Read the model definition and answer for the solid it produces. Units are mm, in the model's axes. Coordinates: 2 decimals unless noted, no trailing zeros. Write each loop counter-clockwise with the first axis right and the second up, starting at its lowest first coordinate (ties: lowest second). Pieces come first, ordered by that corner, then holes. Notation, with made-up numbers: (16.5, 72.5) -> (66.5, 72.5) arc R25 cw to (66.5, 106.5) -> close; hole circle Ø5 at (-1, 65.5). An arc over 180 degrees is marked (long way). Write item = value, one per line. Start each with the question number.
1) Section D-D (z = -105) is taken. Determine the outline of the cut face in (x, y), plus the area to 3 significant figures.
2) Find the intervals of material crossed by line 1 along Z through (x, y) = (-8, -2.05); line 2 along X through (y, z) = (-4.5, -12); line 3 along Z through (x, y) = (-124, -2.65), in increasing order. Write a range as from..to.
3) Section C-C (z = 33.5) is taken. Determine the outline of the cut face in (x, y).
4) Section B-B (z = -54.5) is taken. Determine the outline of the cut face in (x, y), plus the area to 3 significant figures.
5) Flat-ended cylindrical pins translate along their axes: pin 1 Ø1 at (x, y) = (-46, -2.5) entering from +Z; pin 2 Ø1 at (y, z) = (-3, -18) entering from -X. Find the tip coordinate at first contact, or state that the pin passes through.
6) Section A-A (y = -2.7) is taken. Count the separate pieces of the cut face and the enclosed holes in it, plus the area to 3 significant figures.
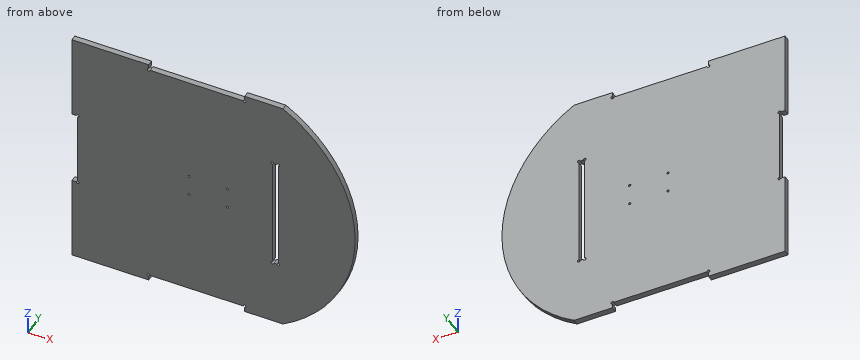
from build123d import *

# Parameters (mm, degrees)
BOSS_EXTRUDE1_DEPTH       = 6
M2_CLEARANCE_HOLE1_D      = 2.4
CUT_EXTRUDE1_REACH        = 212.276
SKETCH4_W                 = 6.1
SKETCH4_H                 = 120.1
SKETCH4_W_2               = 100.1
SKETCH4_H_2               = 6.1
SKETCH4_H_3               = 80.1
F_3_0MM_DOWEL_HOLE1_D     = 3
F_3_0MM_DOWEL_HOLE1_DEPTH = 6


with BuildPart() as part:
    # Sketch1 → Boss-Extrude1 (new body)
    with BuildSketch(Plane(origin=(0, 0, 0), x_dir=(1, 0, 0), z_dir=(0, 1, 0))):
        with BuildLine():
            Line((-130, 130), (90, 130))
            ThreePointArc((90, 130), (165.166852265, 0), (90, -130))
            Line((90, -130), (-130, -130))
            Line((-130, -130), (-130, 130))
        make_face()
    extrude(amount=-BOSS_EXTRUDE1_DEPTH)

    # M2 Clearance Hole1 (through all)
    with Locations(Plane(origin=(0, -6, 0), x_dir=(-1, 0, 0), z_dir=(0, -1, 0))):
        with Locations((-32, -11), (-32, 11), (8, -11), (8, 11)):
            Hole(M2_CLEARANCE_HOLE1_D / 2)

    # Sketch4 → Cut-Extrude1 (cut, up to next)
    with BuildSketch(Plane.XZ.offset(6), mode=Mode.PRIVATE) as cut_extrude1_sk1:
        with Locations((82, 0)):
            Rectangle(SKETCH4_W, SKETCH4_H)
    cut_extrude1_tool1 = extrude(cut_extrude1_sk1.sketch, amount=-CUT_EXTRUDE1_REACH, mode=Mode.PRIVATE) & part.part
    # Sketch4 → Cut-Extrude1 (cut, up to next)
    with BuildSketch(Plane.XZ.offset(6), mode=Mode.PRIVATE) as cut_extrude1_sk2:
        with Locations((0, -127)):
            Rectangle(SKETCH4_W_2, SKETCH4_H_2)
    cut_extrude1_tool2 = extrude(cut_extrude1_sk2.sketch, amount=-CUT_EXTRUDE1_REACH, mode=Mode.PRIVATE) & part.part
    # Sketch4 → Cut-Extrude1 (cut, up to next)
    with BuildSketch(Plane.XZ.offset(6), mode=Mode.PRIVATE) as cut_extrude1_sk3:
        with Locations((0, 127)):
            Rectangle(SKETCH4_W_2, SKETCH4_H_2)
    cut_extrude1_tool3 = extrude(cut_extrude1_sk3.sketch, amount=-CUT_EXTRUDE1_REACH, mode=Mode.PRIVATE) & part.part
    # Sketch4 → Cut-Extrude1 (cut, up to next)
    with BuildSketch(Plane.XZ.offset(6), mode=Mode.PRIVATE) as cut_extrude1_sk4:
        with Locations((-127, 0)):
            Rectangle(SKETCH4_W, SKETCH4_H_3)
    cut_extrude1_tool4 = extrude(cut_extrude1_sk4.sketch, amount=-CUT_EXTRUDE1_REACH, mode=Mode.PRIVATE) & part.part
    add(cut_extrude1_tool1.solids().sort_by_distance((82, -6, 0))[0], mode=Mode.SUBTRACT)
    add(cut_extrude1_tool2.solids().sort_by_distance((0, -6, -127))[0], mode=Mode.SUBTRACT)
    add(cut_extrude1_tool3.solids().sort_by_distance((0, -6, 127))[0], mode=Mode.SUBTRACT)
    add(cut_extrude1_tool4.solids().sort_by_distance((-127, -6, 0))[0], mode=Mode.SUBTRACT)

    # Ø3.0mm Dowel Hole1
    with Locations(Plane(origin=(0, -6, 0), x_dir=(-1, 0, 0), z_dir=(0, -1, 0))):
        with Locations((-85, 60), (-79, 60), (-78.95, -60.05), (-85, -60), (124, 40), (123.95, -40.05), (50.05, -123.95), (-50, -124), (-50.05, 123.95), (50.05, 123.95)):
            Hole(F_3_0MM_DOWEL_HOLE1_D / 2, depth=F_3_0MM_DOWEL_HOLE1_DEPTH)


solid = part.part
Answer key:
q1.outline = (-130, -6) -> (122.29, -6) -> (122.29, 0) -> (-130, 0) -> close
q1.area = 1,510 mm^2
q2.line_1 = -123.95..-12.2, -9.8..9.8, 12.2..123.95
q2.line_2 = -123.95..-8.66, -7.34..31.34, 32.66..78.95, 85.05..164.69
q2.line_3 = -130..-41.5, 41.55..130
q3.outline = (-123.95, -6) -> (78.95, -6) -> (78.95, 0) -> (-123.95, 0) -> close; (85.05, -6) -> (161.38, -6) -> (161.38, 0) -> (85.05, 0) -> close
q4.outline = (-130, -6) -> (78.95, -6) -> (78.95, 0) -> (-130, 0) -> close; (85.05, -6) -> (154.92, -6) -> (154.92, 0) -> (85.05, 0) -> close
q4.area = 1,670 mm^2
q5.pin_1 = 123.95
q5.pin_2 = -123.95
q6.separate_pieces = 1
q6.enclosed_holes = 5
q6.area = 68,600 mm^2
